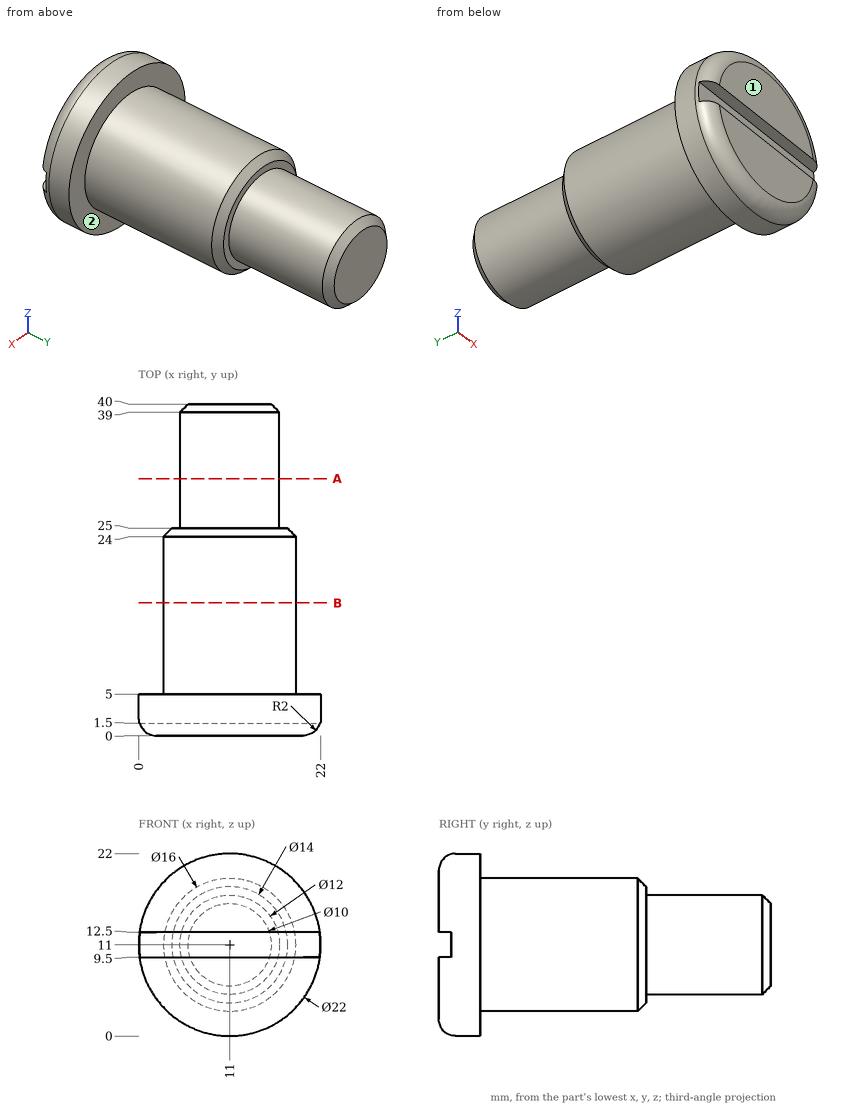
The figure shows three views and two pictorial views of one solid part (mm, origin at its lowest corner). Answer the questions. A direction names the side the tool comes from. Round coordinates to 2 decimals unless told otherwise and drop trailing zeros. Order: outer loops, then holes, each group sorted by start corner. A loop starts at its lowest first (then second) coordinate and runs counter-clockwise, first axis right, second up. Notation, with made-up numbers: (68.25, 53.5) - (123.25, 53.5) arc R26 ccw to (123.25, 81.5) - close; hole circle Ø7 at (78.5, 70.5). An arc over 180 degrees is marked (long way). Write item = value, one per line. Start each with the question number.
1) For the marked faces 1 and 2, determine the directions among +Z, -Z, +X, -X, +Y, -Y from which every point of the face is accessible in a straight line to the end or side of a thin tool.
2) Given pin 1 (5 mm diameter, centred on y = 19, z = 13, fed in from +X); pin 2 (0.5 mm diameter, centred on x = 15.5, y = 0.5, fed in from +Z); pin 3 (1.5 mm diameter, centred on x = 5, z = 6.5, fed in from +Y), each flat-ended and moving along its own axis, determine where each tip first touches the part or whether it passes through.
3) Section B-B, the plane y = 16 is taken. Write down the section's boundary in (x, z), plus the area to 3 significant figures.
4) Straight lines are drawn through the part: L1, parallel to X at y = 11, z = 4.75; L2, parallel to Y at x = 16.5, z = 17.5; L3, parallel to Y at x = 8.5, z = 11.5. For each, find the intervals that lie inside material, in ascending order.
5) Section A-A, the plane y = 31 is taken. Write down the section's boundary in (x, z).
Results list:
q1.face_1 = +Z, -Z, +X, -X, -Y
q1.face_2 = +Y
q2.pin_1 = 19
q2.pin_2 = 20.58
q2.pin_3 = 25
q3.outline = circle Ø16 at (11, 11)
q3.area = 201 mm^2
q4.L1 = 6.01 to 15.99
q4.L2 = 0 to 5
q4.L3 = 1.5 to 40
q5.outline = circle Ø12 at (11, 11)
